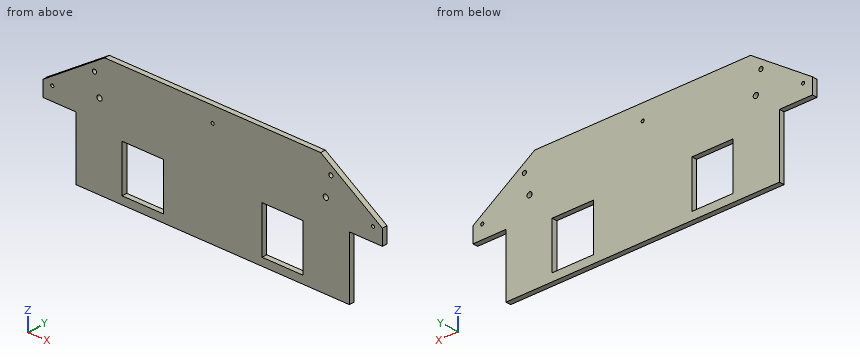
from build123d import *

# Parameters (mm, degrees)
ESQUISSE1_W             = 330
ESQUISSE1_H             = 250
EXTRUSION1_DEPTH        = 5
ESQUISSE2_W             = 32
ESQUISSE2_H             = 60
ENL_V_MAT_EXTRU_1_DEPTH = 362.087798138
ESQUISSE4_W             = 40
ESQUISSE4_H             = 45
ENL_V_MAT_EXTRU_2_DEPTH = 362.087798138
CHANFREIN1_SIZE         = 15
ESQUISSE5_W             = 330
ESQUISSE5_H             = 5
ENL_V_MAT_EXTRU_3_DEPTH = 15
ENL_V_MAT_EXTRU_5_DEPTH = 352.563639113
ESQUISSE9_R             = 17.5
ENL_V_MAT_EXTRU_6_DEPTH = 352.563639255
SKETCH1_R               = 2
EXTRUDE1_DEPTH          = 5
ESQUISSE10_R            = 2.5
ESQUISSE10_R_2          = 1.5
ENL_V_MAT_EXTRU_7_DEPTH = 6


with BuildPart() as part:
    # Esquisse1 → Extrusion1 (new body)
    with BuildSketch(Plane(origin=(0, 0, 0), x_dir=(1, 0, 0), z_dir=(0, 1, 0))):
        with Locations((110.175955056, 108.746853933)):
            Rectangle(ESQUISSE1_W, ESQUISSE1_H)
    extrude(amount=EXTRUSION1_DEPTH)

    # Esquisse2 → Enlèv. mat.-Extru.1 (cut, through all)
    with BuildSketch(Plane(origin=(0, 5, 0), x_dir=(-1, 0, 0), z_dir=(0, 1, 0))):
        with Locations((38.824044944, -188.746853933)):
            Rectangle(ESQUISSE2_W, ESQUISSE2_H)
        with Locations((-259.175955056, -188.746853933)):
            Rectangle(ESQUISSE2_W, ESQUISSE2_H)
    extrude(amount=-ENL_V_MAT_EXTRU_1_DEPTH, mode=Mode.SUBTRACT)

    # Esquisse4 → Enlèv. mat.-Extru.2 (cut, through all)
    with BuildSketch(Plane(origin=(0, 5, 0), x_dir=(-1, 0, 0), z_dir=(0, 1, 0))):
        with Locations((-178.175955056, -188.746853933)):
            Rectangle(ESQUISSE4_W, ESQUISSE4_H)
        with Locations((-42.175955056, -188.746853933)):
            Rectangle(ESQUISSE4_W, ESQUISSE4_H)
    extrude(amount=-ENL_V_MAT_EXTRU_2_DEPTH, mode=Mode.SUBTRACT)

    # Chanfrein1
    chanfrein1_edges = [part.edges().sort_by_distance(p)[0] for p in [
        (275.175955056, 2.5, 16.253146067),
        (-54.824044944, 2.5, 16.253146067),
    ]]
    chamfer(chanfrein1_edges, length=CHANFREIN1_SIZE)

    # Esquisse5 → Enlèv. mat.-Extru.3 (cut)
    with BuildSketch(Plane(origin=(0, 0, -233.746853933), x_dir=(-1, 0, 0), z_dir=(0, 0, -1))):
        with Locations((-110.175955056, 2.5)):
            Rectangle(ESQUISSE5_W, ESQUISSE5_H)
    extrude(amount=-ENL_V_MAT_EXTRU_3_DEPTH, mode=Mode.SUBTRACT)

    # Esquisse8 → Enlèv. mat.-Extru.5 (cut, through all)
    with BuildSketch(Plane(origin=(0, 5, 0), x_dir=(-1, 0, 0), z_dir=(0, 1, 0))):
        with BuildLine():
            Line((-129.175955056, -33.746853933), (-195.175955056, 16.253146067))
            Line((-195.175955056, 16.253146067), (-25.175955056, 16.253146067))
            Line((-25.175955056, 16.253146067), (-61.175955056, -33.746853933))
            add(Edge.make_bspline(
                [(-95.175955056, -83.746853933), (-72.555573237, -83.746853933), (-61.175955056, -53.90180921), (-61.175955056, -33.746853933)],
                knots=[0, 0, 0, 0, 1, 1, 1, 1], degree=3))
            add(Edge.make_bspline(
                [(-95.175955056, -83.746853933), (-117.796336875, -83.746853933), (-129.175955056, -53.90180921), (-129.175955056, -33.746853933)],
                knots=[0, 0, 0, 0, 1, 1, 1, 1], degree=3))
        make_face()
    extrude(amount=-ENL_V_MAT_EXTRU_5_DEPTH, mode=Mode.SUBTRACT)

    # Esquisse9 → Enlèv. mat.-Extru.6 (cut, through all)
    with BuildSketch(Plane(origin=(0, 5, 0), x_dir=(-1, 0, 0), z_dir=(0, 1, 0))):
        with Locations(Location((-205.175955056, -33.746853933, 0), (0, 0, 90))):
            Circle(ESQUISSE9_R)
        with Locations(Location((-15.175955056, -33.746853933, 0), (0, 0, 90))):
            Circle(ESQUISSE9_R)
    extrude(amount=-ENL_V_MAT_EXTRU_6_DEPTH, mode=Mode.SUBTRACT)

    # Sketch1 → Extrude1 (cut)
    with BuildSketch(Plane.XZ):
        with Locations(Location((-4.824044944, -118.746853933, 0), (0, 0, 270))):
            Circle(SKETCH1_R)
        with Locations(Location((225.175955056, -118.746853933, 0), (0, 0, 90))):
            Circle(SKETCH1_R)
        Polygon((-54.824044944, -143.746853933), (5.175955056, -103.746853933), (215.175955056, -103.746853933), (275.175955056, -143.746853933), (275.175955056, 16.253146067), (-54.824044944, 16.253146067), align=None)
    extrude(amount=-EXTRUDE1_DEPTH, mode=Mode.SUBTRACT)

    # Esquisse10 → Enlèv. mat.-Extru.7 (cut)
    with BuildSketch(Plane.XZ):
        with Locations(Location((0.175955056, -138.746853933, 0), (0, 0, 270))):
            Circle(ESQUISSE10_R)
        with Locations(Location((220.175955056, -138.746853933, 0), (0, 0, 90))):
            Circle(ESQUISSE10_R)
        with Locations(Location((-45.824044944, -145.746853933, 0), (0, 0, 270))):
            Circle(ESQUISSE10_R_2)
        with Locations(Location((266.175955056, -145.746853933, 0), (0, 0, 90))):
            Circle(ESQUISSE10_R_2)
        with Locations(Location((110.175955056, -118.746853933, 0), (0, 0, 270))):
            Circle(ESQUISSE10_R_2)
    extrude(amount=-ENL_V_MAT_EXTRU_7_DEPTH, mode=Mode.SUBTRACT)


solid = part.part
Verification items for the finished model (mm, model axes). Give positions to 0.01 mm unless a question says otherwise; leave off trailing zeros. Write each loop counter-clockwise with the first axis right and the second up, starting at its lowest first coordinate (ties: lowest second). Pieces come first, ordered by that corner, then holes. Notation, with made-up numbers: M 76,59.25 L 114,59.25 A37 ccw 114,96.25 Z; hole C 39,75 d1. An arc over 180 degrees is marked long. Write item = value, one per line.
(1) Sectioned sample at A-A (z = -207). Record the cut outline in (x, y), then the cut area to 3 significant figures.
Found:
outline = M -22.82,0 L 22.18,0 L 22.18,5 L -22.82,5 Z; M 62.18,0 L 158.18,0 L 158.18,5 L 62.18,5 Z; M 198.18,0 L 243.18,0 L 243.18,5 L 198.18,5 Z
area = 930 mm2
(2) Material ranges on line 1 (X direction, y = 3.8, z = -201); line 2 (X direction, y = 1.45, z = -118.5); line 3 (X direction, y = 2.15, z = -136.5), recorded low to high.
Found:
line_1 = -22.82 to 22.18, 62.18 to 158.18, 198.18 to 243.18
line_2 = -16.95 to -6.81, -2.84 to 108.7, 111.66 to 223.19, 227.16 to 237.31
line_3 = -43.95 to -0.92, 1.27 to 219.08, 221.27 to 264.31
(3) Sectioned sample at B-B (y = 3.75). Give the number of separate pieces and of enclosed holes in the cut face, then the cut area to 3 significant figures.
Found:
separate_pieces = 1
enclosed_holes = 9
area = 28,000 mm2
(4) Sectioned sample at D-D (x = 230). Record the cut outline in (y, z).
Found:
outline = M 0,-218.75 L 5,-218.75 L 5,-113.63 L 0,-113.63 Z
(5) Sectioned sample at C-C (x = -18). Record the cut outline in (y, z).
Found:
outline = M 0,-218.75 L 5,-218.75 L 5,-119.2 L 0,-119.2 Z
(6) Go/stop test with flat-tipped pins: pin 1 Ø1 at (y, z) = (2, -204) entering from -X; pin 2 Ø2.5 at (x, y) = (266, 2.5) entering from -Z; pin 3 Ø3 at (x, y) = (224, 2) entering from +Z. Record where each tip stops, or that it passes through.
Found:
pin_1 = -22.82
pin_2 = -158.75
pin_3 = -108.63
